from build123d import *

# Parameters (mm, degrees)
BOSS_EXTRUDE2_DEPTH = 10
CUT_EXTRUDE1_REACH  = 134.798
CUT_EXTRUDE2_REACH  = 134.58


with BuildPart() as part:
    # Sketch1 → Boss-Extrude2 (new body)
    with BuildSketch(Plane(origin=(0, 0, 0), x_dir=(1, 0, 0), z_dir=(0, 1, 0))):
        with BuildLine():
            Line((-20.75, 0), (-12.75, 0))
            Line((-12.75, 0), (-12.75, 8.502685995))
            ThreePointArc((-12.75, 8.502685995), (-16.75, 12.502685995), (-12.75, 16.502685995))
            Line((-12.75, 16.502685995), (-12.75, 86.85))
            ThreePointArc((-12.75, 86.85), (-16.749999279, 90.852402374), (-12.745195252, 94.849997114))
            ThreePointArc((-12.745195252, 94.849997114), (0, 107.25), (12.745195252, 94.849997114))
            ThreePointArc((12.745195252, 94.849997114), (16.749999279, 90.852402374), (12.75, 86.85))
            Line((12.75, 86.85), (12.75, 16.502685995))
            ThreePointArc((12.75, 16.502685995), (16.75, 12.502685995), (12.75, 8.502685995))
            Line((12.75, 8.502685995), (12.75, 0))
            Line((12.75, 0), (20.75, 0))
            Line((20.75, 0), (20.75, 105))
            ThreePointArc((20.75, 105), (0, 125.75), (-20.75, 105))
            Line((-20.75, 105), (-20.75, 0))
        make_face()
    extrude(amount=BOSS_EXTRUDE2_DEPTH)

    # Cut-Extrude1: up to this face of the body (flat: up to its plane)
    cut_extrude1_end = Plane(part.part.faces().sort_by_distance((-20.75, 5, -52.5))[0])
    # Sketch2 → Cut-Extrude1 (cut, up to the picked face)
    with BuildSketch(Plane(origin=(20.75, 0, 0), x_dir=(0, 0, -1), z_dir=(1, 0, 0)), mode=Mode.PRIVATE) as cut_extrude1_sk1:
        with BuildLine():
            Line((0, 10), (0, 6))
            add(Edge.make_bspline(
                [(0, 6), (20.380438902, 6.489130534), (49.317340974, 6.513055303), (79.861692853, 6.559373615), (105, 6.320685747)],
                knots=[0, 0, 0, 0, 0, 0.815217556, 0.815217556, 0.815217556, 0.815217556, 0.815217556], degree=4))
            Line((105, 6.320685747), (105, 10))
            Line((105, 10), (0, 10))
        make_face()
    cut_extrude1_tool1 = split(extrude(cut_extrude1_sk1.sketch, amount=-CUT_EXTRUDE1_REACH, mode=Mode.PRIVATE), bisect_by=cut_extrude1_end, keep=Keep.BOTH, mode=Mode.PRIVATE)
    # Sketch2 → Cut-Extrude1 (cut, up to the picked face)
    with BuildSketch(Plane(origin=(20.75, 0, 0), x_dir=(0, 0, -1), z_dir=(1, 0, 0)), mode=Mode.PRIVATE) as cut_extrude1_sk2:
        with BuildLine():
            Line((105, 10), (105, 6.320685747))
            add(Edge.make_bspline(
                [(105, 6.320685747), (110.698010054, 6.266583223), (116.118270151, 6.197837747), (121.179103999, 6.110869466), (125.798665098, 6)],
                knots=[0.815217556, 0.815217556, 0.815217556, 0.815217556, 0.815217556, 1, 1, 1, 1, 1], degree=4))
            Line((125.798665098, 6), (125.75, 10))
            Line((125.75, 10), (105, 10))
        make_face()
    cut_extrude1_tool2 = split(extrude(cut_extrude1_sk2.sketch, amount=-CUT_EXTRUDE1_REACH, mode=Mode.PRIVATE), bisect_by=cut_extrude1_end, keep=Keep.BOTH, mode=Mode.PRIVATE)
    add(cut_extrude1_tool1.solids().sort_by(Axis((20.75, 8.191223, -51.89052), (-1, 0, 0)))[0], mode=Mode.SUBTRACT)
    add(cut_extrude1_tool2.solids().sort_by(Axis((20.75, 8.09056, -115.529992), (-1, 0, 0)))[0], mode=Mode.SUBTRACT)

    # Cut-Extrude2: up to this face of the body (flat: up to its plane)
    cut_extrude2_end = Plane(part.part.faces().sort_by_distance((-20.75, 3.194161628, -52.844890182))[0])
    # Sketch3 → Cut-Extrude2 (cut, up to the picked face)
    with BuildSketch(Plane(origin=(20.75, 0, 0), x_dir=(0, 0, -1), z_dir=(1, 0, 0)), mode=Mode.PRIVATE) as cut_extrude2_sk1:
        with BuildLine():
            Line((0, 0), (0, 2))
            add(Edge.make_bspline(
                [(0, 2), (20.957324469, 2.318248008), (62.875, 4.681751992), (104.792675531, 2.318248008), (125.75, 2)],
                knots=[0, 0, 0, 0, 0.5, 1, 1, 1, 1], degree=3))
            Line((125.75, 2), (125.75, 0))
            Line((125.75, 0), (0, 0))
        make_face()
    cut_extrude2_tool1 = split(extrude(cut_extrude2_sk1.sketch, amount=-CUT_EXTRUDE2_REACH, mode=Mode.PRIVATE), bisect_by=cut_extrude2_end, keep=Keep.BOTH, mode=Mode.PRIVATE)
    add(cut_extrude2_tool1.solids().sort_by(Axis((20.75, 1.458103, -62.875), (-1, 0, 0)))[0], mode=Mode.SUBTRACT)


solid = part.part
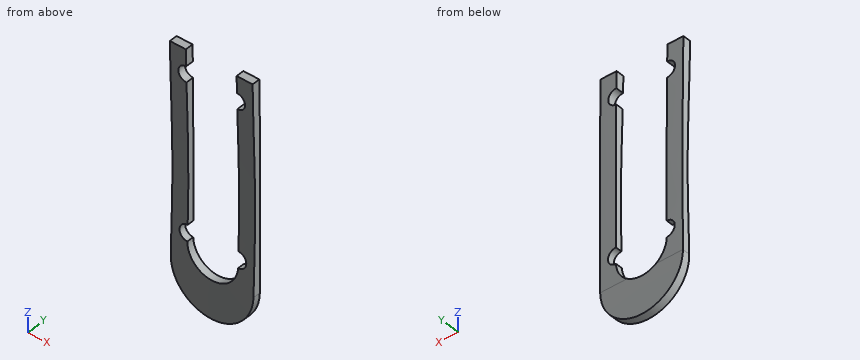
Work out the finished part from the listing and answer in its coordinate system (mm). Give positions to 0.01 mm unless a question says otherwise; leave off trailing zeros. Loops run counter-clockwise (first coordinate to the right, second up) from the corner with the lowest first, then second, coordinate; pieces in that order, holes last. Notation, with made-up numbers: (61.5, 34) - (79.5, 34) arc R10 ccw to (79.5, 42) - close; hole circle Ø4 at (4, 1). An arc over 180 degrees is marked (long way). Answer in a Markdown table with one row per item.
(1) Consider L1, parallel to X at y = 5.3, z = -45.5; L2, parallel to X at y = 6, z = -97; L3, parallel to Y at x = 18, z = -110. Determine where each line is inside the solid, lowest interval first. Write a range as [from, to].
Results list:
| item | result |
|---|---|
| L1 | x = [-20.75, -12.75], [12.75, 20.75] |
| L2 | x = [-20.75, -12.5], [12.5, 20.75] |
| L3 | y = [2.37, 6.27] |
(2) Section B-B (x = -15) is taken. State how many separate pieces and enclosed holes the cut face has, and give its area (3 significant figures).
Results list:
| item | result |
|---|---|
| separate pieces | 3 |
| enclosed holes | 0 |
| area | 368 mm² |
(3) Flat-ended cylindrical pins translate along their axes: pin 1 Ø2 at (y, z) = (5.5, -112) entering from +X; pin 2 Ø1.5 at (x, y) = (-1.5, 3) entering from +Z; pin 3 Ø1 at (x, z) = (3.5, -111) entering from -Y. Find the tip coordinate at first contact, or state that the pin passes through.
Results list:
| item | result |
|---|---|
| pin 1 | stops at x = 19.86 |
| pin 2 | stops at z = -107.05 |
| pin 3 | stops at y = 2.33 |
(4) Section A-A (y = 4.35) is taken. Give the vertices of the cut face in (x, z).
Results list:
| item | result |
|---|---|
| outline | (-20.75, -105) arc R20.75 ccw to (20.75, -105) - (20.75, 0) - (12.75, 0) - (12.75, -8.5) arc R4 cw to (12.75, -16.5) - (12.75, -86.85) arc R4 cw to (12.75, -94.85) arc R12.75 cw to (-12.75, -94.85) arc R4 cw to (-12.75, -86.85) - (-12.75, -16.5) arc R4 cw to (-12.75, -8.5) - (-12.75, 0) - (-20.75, 0) - close |
